from build123d import *

# Parameters (mm, degrees)
SKETCH_W        = 39
SKETCH_H        = 43
SKETCH_R        = 7
SKETCH_R_2      = 1.7
PAD_DEPTH       = 3.6
SKETCH001_R     = 2.95
POCKET_DEPTH    = 1.6
SKETCH002_W     = 10
SKETCH002_H     = 8.4
PAD001_DEPTH    = 8
SKETCH003_R     = 1.7
POCKET001_DEPTH = 33.001
POCKET002_DEPTH = 1.5
PAD002_DEPTH    = 12.5


with BuildPart() as part:
    # Sketch → Pad (new body)
    with BuildSketch(Plane.XY):
        with Locations((2, 0)):
            Rectangle(SKETCH_W, SKETCH_H)
        Circle(SKETCH_R, mode=Mode.SUBTRACT)
        with Locations((-15.5, 15.5)):
            Circle(SKETCH_R_2, mode=Mode.SUBTRACT)
        with Locations((15.5, 15.5)):
            Circle(SKETCH_R_2, mode=Mode.SUBTRACT)
        with Locations((15.5, -15.5)):
            Circle(SKETCH_R_2, mode=Mode.SUBTRACT)
        with Locations((-15.5, -15.5)):
            Circle(SKETCH_R_2, mode=Mode.SUBTRACT)
    extrude(amount=PAD_DEPTH)

    # Sketch001 (on Face11 of Pad) → Pocket (cut)
    with BuildSketch(Plane.XY.offset(3.6)):
        with Locations((-15.5, -15.5)):
            Circle(SKETCH001_R)
        with Locations((15.5, -15.5)):
            Circle(SKETCH001_R)
        with Locations((15.5, 15.5)):
            Circle(SKETCH001_R)
        with Locations((-15.5, 15.5)):
            Circle(SKETCH001_R)
    extrude(amount=-POCKET_DEPTH, mode=Mode.SUBTRACT)

    # Sketch002 (on Face5 of Pocket) → Pad001 (join)
    with BuildSketch(Plane.XY.offset(3.6)):
        with Locations((16.5, -7.3)):
            Rectangle(SKETCH002_W, SKETCH002_H)
    extrude(amount=PAD001_DEPTH)

    # Sketch003 (on Face15 of Pad001) → Pocket001 (cut, through all)
    with BuildSketch(Plane.XZ.offset(11.5)):
        with Locations((16.5, 7.6)):
            Circle(SKETCH003_R)
    extrude(amount=-POCKET001_DEPTH, mode=Mode.SUBTRACT)

    # Sketch004 (on DatumPlane) → Pocket002 (cut, symmetric)
    with BuildSketch(Plane.XZ.offset(7.3)):
        Polygon((13.598815, 5.925), (16.5, 4.25), (19.401185, 5.925), (19.401185, 15.925), (13.598815, 15.925), align=None)
    extrude(amount=POCKET002_DEPTH, both=True, mode=Mode.SUBTRACT)

    # Sketch005 → Pad002 (join, symmetric)
    with BuildSketch(Plane.XZ):
        Polygon((-14.9, 7.7), (-6.1, 7.7), (-10.5, 2.456284), align=None)
    extrude(amount=PAD002_DEPTH, both=True)


solid = part.part
Part model, mm, in its own coordinate system. A direction names the side the tool comes from. Give positions to 0.01 mm unless a question says otherwise; leave off trailing zeros. Order: outer loops, then holes, each group sorted by start corner. A loop starts at its lowest first (then second) coordinate and runs counter-clockwise, first axis right, second up. Notation, with made-up numbers: (-4, 20) -> (29, 20) arc R19 cw to (29, 43) -> close; hole circle Ø3 at (46, -11). An arc over 180 degrees is marked (long way). Use one line per item in the form item = value.
(1) Drill centre lines: line 1 (Y direction, x = 15.5, z = 1.1); line 2 (X direction, y = 15.5, z = 0.8); line 3 (Y direction, x = 15.5, z = 2.8). Where is each one in solid material? Low to high. Write a range as from..to.
Solution:
line_1 = -21.5..-17.2, -13.8..13.8, 17.2..21.5
line_2 = -17.5..-17.2, -13.8..13.8, 17.2..21.5
line_3 = -21.5..-18.45, -12.55..12.55, 18.45..21.5
(2) Tool access for faces 4 (the face through (17, -17, 2)), 5 (the face through (11.5, -7, 8)), 6 (the face through (15, -11.5, 9)), 7 (the face through (-11, 0, 7.7)): list every direction of +Z, -Z, +X, -X, +Y, -Y with a clear straight run to the whole face (end or side of a thin tool).
Solution:
face_4 = +Z
face_5 = +Z, +Y, -Y
face_6 = +Z, +X, -Y
face_7 = +Z, -X, +Y, -Y
(3) Saw through at D-D (y = 0). Write the cut outline in (x, z).
Solution:
outline = (-17.5, 0) -> (-7, 0) -> (-7, 3.6) -> (-9.54, 3.6) -> (-6.1, 7.7) -> (-14.9, 7.7) -> (-11.46, 3.6) -> (-17.5, 3.6) -> close; (7, 0) -> (21.5, 0) -> (21.5, 3.6) -> (7, 3.6) -> close
(4) Saw through at B-B (x = -15.5). Write the cut outline in (y, z), then the cut area to 3 significant figures.
Solution:
outline = (-21.5, 0) -> (-17.2, 0) -> (-17.2, 2) -> (-18.45, 2) -> (-18.45, 3.6) -> (-21.5, 3.6) -> close; (-13.8, 0) -> (13.8, 0) -> (13.8, 2) -> (12.55, 2) -> (12.55, 3.6) -> (-12.55, 3.6) -> (-12.55, 2) -> (-13.8, 2) -> close; (17.2, 0) -> (21.5, 0) -> (21.5, 3.6) -> (18.45, 3.6) -> (18.45, 2) -> (17.2, 2) -> close
area = 122 mm²
(5) Flat gauge pins, fed straight in: P1, Ø4, axis at x = 16.5, z = 7.6, coming from the -Y side; P2, Ø1.8, axis at x = 14, y = 15.5, coming from the +Z side; P3, Ø22.5, axis at x = 0, y = 0, coming from the +Z side. Where does each tip first touch, or does it go through?
Solution:
P1 = -11.5
P2 = 2
P3 = 7.7
(6) Pull direction Z, two halves, no side cores. Call faces 1 (the face through (18.07, -4.47, 6.95)), 2 (the face through (16, -5.8, 10)), 3 (the face through (17.93, -7.321, 5.076)): +Z half, -Z half, draft (parallel to the pull), parting line (faces both ways), or undercut.
Solution:
face_1 = undercut
face_2 = draft
face_3 = +Z half
(7) Saw through at A-A (y = -15.5). Write the cut outline in (x, z), then the cut area to 3 significant figures.
Solution:
outline = (-17.5, 0) -> (-17.2, 0) -> (-17.2, 2) -> (-17.5, 2) -> close; (-13.8, 0) -> (13.8, 0) -> (13.8, 2) -> (12.55, 2) -> (12.55, 3.6) -> (-12.55, 3.6) -> (-12.55, 2) -> (-13.8, 2) -> close; (17.2, 0) -> (21.5, 0) -> (21.5, 3.6) -> (18.45, 3.6) -> (18.45, 2) -> (17.2, 2) -> close
area = 109 mm²
(8) Saw through at C-C (z = 1.25). Write the cut outline in (x, y).
Solution:
outline = (-17.5, -21.5) -> (21.5, -21.5) -> (21.5, 21.5) -> (-17.5, 21.5) -> close; hole circle Ø3.4 at (-15.5, -15.5); hole circle Ø3.4 at (-15.5, 15.5); hole circle Ø14 at (0, 0); hole circle Ø3.4 at (15.5, -15.5); hole circle Ø3.4 at (15.5, 15.5)
